Input: part model. Units: mm. Frame: model coordinates. A direction names the side the tool comes from. Round coordinates to 2 decimals unless told otherwise and drop trailing zeros. Use one line per item in the form item = value. Start each with the question number.
Q1. Ray query, line 1 along Y through (x, z) = (95.5, 2.8); line 2 along X through (y, z) = (13.5, 3.05). Return the intervals inside material, ascending.
Q2. Access query for faces 4 (the flat face through (97, 9, 2)), 5 (the flat face through (2, 22, 2)), 6 (the flat face through (5, 6, 2)), 7 (the flat face through (95, 17, 2)). Directions: +Z, -Z, +X, -X, +Y, -Y. A direction counts if a zero-diameter tool reaches every point of the face in a straight line with its end or side. Return the directions, or none.
Q3. Mould query, pull axis Y, two halves, no side actions, for faces 1 (the flat face through (97, 13, 2)), 2 (the flat face through (49, 4, 2)), 3 (the flat face through (100, 60, 2)). Classes: pulls with the +Y half, pulls with the -Y half, needs draft (parallel to the pull), parting line crosses it, or undercut.
Q4. First-contact query: P1, Ø1.2, axis at x = 96.5, z = 2, coming from the -Y side; P2, Ø2, axis at y = 6, z = 2.5, coming from the +X side. Flat tips, straight axial feed; report the tip coordinate or a pass-through.
```python
from build123d import *

# Parameters (mm, degrees)
F0_W      = 100
F0_H      = 100
F1_DEPTH  = 4
F2_W      = 5
F2_H      = 22
F3_DEPTH  = 4
F4_W      = 10
F4_H      = 4
F5_DEPTH  = 4
F6_W      = 5
F6_H      = 4
F7_DEPTH  = 4
F8_W      = 5
F8_H      = 4
F9_DEPTH  = 4
F10_W     = 90
F10_H     = 4
F11_DEPTH = 4


with BuildPart() as f1:
    # F0 (on Top) → F1 (new body)
    with BuildSketch(Plane.XY):
        with Locations((50, 50)):
            Rectangle(F0_W, F0_H)
    extrude(amount=F1_DEPTH)

    # F2 (on Top) → F3 (cut)
    with BuildSketch(Plane.XY):
        with Locations((2.5, 11)):
            Rectangle(F2_W, F2_H)
        with Locations((97.5, 11)):
            Rectangle(F2_W, F2_H)
    extrude(amount=F3_DEPTH, mode=Mode.SUBTRACT)

    # F4 (on Top) → F5 (join)
    with BuildSketch(Plane.XY):
        with Locations((0, 11)):
            Rectangle(F4_W, F4_H)
        with Locations((100, 11)):
            Rectangle(F4_W, F4_H)
    extrude(amount=F5_DEPTH)

    # F6 (on Top) → F7 (cut)
    with BuildSketch(Plane.XY):
        with Locations((-2.5, 11)):
            Rectangle(F6_W, F6_H)
    extrude(amount=F7_DEPTH, mode=Mode.SUBTRACT)

    # F8 (on Top) → F9 (cut)
    with BuildSketch(Plane.XY):
        with Locations((102.5, 11)):
            Rectangle(F8_W, F8_H)
    extrude(amount=F9_DEPTH, mode=Mode.SUBTRACT)

    # F10 (on Top) → F11 (cut)
    with BuildSketch(Plane.XY):
        with Locations((50, 2)):
            Rectangle(F10_W, F10_H)
    extrude(amount=F11_DEPTH, mode=Mode.SUBTRACT)


solid = f1.part
```
Results found:
q1.line_1 = 9 to 13, 22 to 100
q1.line_2 = 5 to 95
q2.face_4 = +Z, -Z, +X, -Y
q2.face_5 = +Z, -Z, -X
q2.face_6 = +Z, -Z, -X, -Y
q2.face_7 = +Z, -Z, +X
q3.face_1 = undercut
q3.face_2 = pulls with the -Y half
q3.face_3 = needs draft
q4.P1 = 9
q4.P2 = 95
